Work out the finished part from the listing and answer in its coordinate system (mm). A direction names the side the tool comes from. Coordinates: 2 decimals unless noted, no trailing zeros. Order: outer loops, then holes, each group sorted by start corner. A loop starts at its lowest first (then second) coordinate and runs counter-clockwise, first axis right, second up. Notation, with made-up numbers: (31, 79.5) -> (81, 79.5) arc R26 ccw to (81, 115.5) -> close; hole circle Ø9 at (35.25, -12.5). An arc over 180 degrees is marked (long way). Write item = value, one per line. Start each with the question number.
Q1. Flat-ended cylindrical pins translate along their axes: pin 1 (1 mm diameter, centred on x = 8, y = 16, fed in from -Z); pin 2 (5 mm diameter, centred on x = 11.5, z = 4, fed in from +Y); pin 3 (6 mm diameter, centred on x = -13.5, z = 59, fed in from -Y). Find the tip coordinate at first contact, or state that the pin passes through.
Q2. Straight lines are drawn through the part: L1, parallel to X at y = 0, z = 57; L2, parallel to Z at x = -9, y = -4. For each, find the intervals that lie inside material, in ascending order. Write a range as from..to.
Q3. For a pull along Y with two mould halves and no side action, classify faces 3 (the flat face through (0, 0, 80)), 4 (the cylindrical face through (20.03, -6.31, 40.6)), 5 (the flat face through (0, 0, 81.8)) as +Y half, -Y half, draft (parallel to the pull), parting line (faces both ways), or undercut.
Q4. Which of the six approach directions +Z, -Z, +X, -X, +Y, -Y give full straight-line access (tool end or side, diameter ignored) to faces 1 (the flat face through (8, 19, -8)), 2 (the cylindrical face through (8.767, 16.856, 38.454))?
Q5. The part is cut by section A-A, the plane z = 39. Determine the outline of the cut face in (x, y).
Autodesk Inventor part; units mm, degrees
ref_plane "YZ Plane" through (0, 0, 0) normal (1, 0, 0) x (0, 1, 0)
ref_plane "XZ Plane" through (0, 0, 0) normal (0, 1, 0) x (-1, 0, 0)
ref_plane "XY Plane" through (0, 0, 0) normal (0, 0, 1) x (1, 0, 0)
sketch "Skizze1" plane through (0, 0, 0) normal (0, 0, 1) x (1, 0, 0)
  circle A0 centre (0, 0) radius 19
  circle A1 centre (0, 0) radius 21
  dimension "d0" = 38
  dimension "d1" = 2
extrude "Extrusion1" add sketch "Skizze1" along normal blind 80
sketch "Skizze2" plane through (0, 0, 80) normal (0, 0, 1) x (1, 0, 0)
  circle A0 centre (0, 0) radius 21
extrude "Extrusion2" add sketch "Skizze2" along normal blind 1.8
fillet "Rundung1" radius 2 2 edges at (-21, 0, 81.8) (-19, 0, 80)
sketch "Skizze3" plane through (0, 0, 0) normal (1, 0, 0) x (0, 1, 0)
  line L0 (-21, 0) -> (21, 0)
  line L1 (21, 0) -> (23, -2.5) construction
  line L2 (23, -2.5) -> (21, -4) construction
  line L3 (21, -4) -> (21, -8) construction
  spline S0 degree 3 poles (21, 0) (23, -2.5) (21, -4) (21, -8) knots 1 1 1 1 2 2 2 2
  spline S1 degree 2 poles (19, 0) (21, -2.5) (19, -5) knots 0 0 0 1 1 1
  line L4 (19, -5) -> (19, -8)
  line L5 (19, -8) -> (21, -8)
  line L6 (21, 0) -> (19, 0)
  line L7 (21, 0) -> (21, 79.8)
  line L8 (21, 0) -> (21, 79.8)
  line L9 (0, -25.6969) -> (0, 97.3828)
  point P0 (0, 0)
  point P1 (20, -2.5)
  dimension "d7" = 2
  dimension "d8" = 2
  dimension "d9" = 8
  dimension "d10" = 1
  dimension "d11" = 2.5
  dimension "d12" = 5
  dimension "d13" = 4
revolve "Umdrehung1" add sketch "Skizze3" angle 360 about axis through (0, 0, -10) along (0, 0, 1)
fillet "Rundung2" radius 10 1 edges at (14.8492, 14.8492, 0)
chamfer "Fase1" distance 1 angle 45 1 edges at (0, -19, -8)
equation "\"G_L\" = 0"
equation "\"G_H\" = 0"
equation "\"G_B\" = 0"
properties part number "Löffelbox_oben" material "GEDA Stahl"
Model answer:
q1.pin_1 = 79.44
q1.pin_2 = 18.97
q1.pin_3 = -18.19
q2.L1 = -21..-19, 19..21
q2.L2 = 80..81.8
q3.face_3 = undercut
q3.face_4 = parting line
q3.face_5 = draft
q4.face_1 = -Z, +X, -X, +Y, -Y
q4.face_2 = -Z
q5.outline = circle Ø42 at (0, 0); hole circle Ø38 at (0, 0)
